from build123d import *

# Parameters (mm, degrees)
CONE_ROLL_ANGLE    = 90
CONE001_ROLL_ANGLE = 90


with BuildPart() as cone:
    # Cone → Cone (revolve)
    with BuildSketch(Plane.XZ):
        Polygon((0, 0), (1.5, 0), (1.75, 2), (0, 2), align=None)
    revolve(axis=Axis((0, 0, 0), (0, 0, 1)))


with BuildPart() as cone_1:
    # Cone roll: moved
    add(cone.part.rotate(Axis((0, 0, 0), (1, 0, 0)), CONE_ROLL_ANGLE))


with BuildPart() as cone_2:
    # Cone placement: moved
    add(cone_1.part.moved(Location((0, 12, 26.35))))


with BuildPart() as switch_cap:
    # Cone001 → Cone001 (revolve)
    with BuildSketch(Plane.XZ):
        Polygon((0, 0), (2.5, 0), (2.75, 4), (0, 4), align=None)
    revolve(axis=Axis((0, 0, 0), (0, 0, 1)))


with BuildPart() as switch_cap_1:
    # Cone001 roll: moved
    add(switch_cap.part.rotate(Axis((0, 0, 0), (1, 0, 0)), CONE001_ROLL_ANGLE))


with BuildPart() as switch_cap_2:
    # Cone001 placement: moved
    add(switch_cap_1.part.moved(Location((0, 14, 26.35))))

    # Cut012: cut Cone
    add(cone_2.part, mode=Mode.SUBTRACT)


solid = switch_cap_2.part
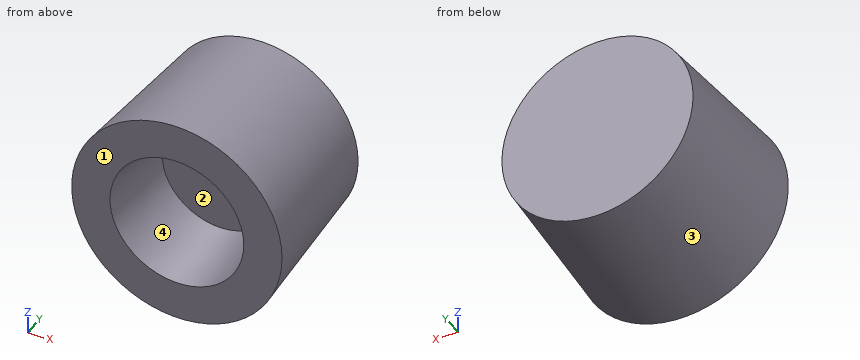
Verification items for the finished model (mm, model axes). Face numbers are marked on the shaded views. Give positions to 0.01 mm unless a question says otherwise; leave off trailing zeros. Loops run counter-clockwise (first coordinate to the right, second up) from the corner with the lowest first, then second, coordinate; pieces in that order, holes last. Notation, with made-up numbers: (33, -31.5) - (81, -31.5) arc R33 cw to (81, 0.5) - close; hole circle Ø3 at (81, 33). An arc over 180 degrees is marked (long way). Write item = value, one per line. Start each with the question number.
Q1. Cross-section at D-D, the plane y = 13.6. Enter the section's corners in (x, z) (3 decimals).
Q2. Cross-section at B-B, the plane z = 26.35. Enter the section's corners in (x, y), and give its area (3 significant figures).
Q3. Cross-section at A-A, the plane x = 0. Enter the section's corners in (y, z).
Q4. Mould release check, pull along X, two halves, no side actions. Record for the marked faces 1, 2, 3 and 4: released by +X, released by -X, zero draft, split by the parting line, or undercut.
Q5. Depth check by flat-ended pin: P1, Ø2, axis at y = 10.5, z = 27.5, coming from the +X side. Enter the tip coordinate at first touch or a pass-through.
Q6. Thickness scan on line 1 (Y direction, x = 0.55, z = 27); line 2 (Z direction, x = 0.4, y = 10.55); line 3 (X direction, y = 10.9, z = 27.65). Record the ranges inside material, lowest first.
Answer key:
q1.outline = circle Ø5.05 at (0, 26.35)
q2.outline = (-2.75, 10) - (-1.75, 10) - (-1.5, 12) - (1.5, 12) - (1.75, 10) - (2.75, 10) - (2.5, 14) - (-2.5, 14) - close
q2.area = 14.5 mm^2
q3.outline = (10, 23.6) - (14, 23.85) - (14, 28.85) - (10, 29.1) - (10, 28.1) - (12, 27.85) - (12, 24.85) - (10, 24.6) - close
q4.face_1 = zero draft
q4.face_2 = undercut
q4.face_3 = split by the parting line
q4.face_4 = undercut
q5.P1 = 2.74
q6.line_1 = 12 to 14
q6.line_2 = 23.66 to 24.72, 27.98 to 29.04
q6.line_3 = -2.36 to -1, 1 to 2.36
